```python
from build123d import *

# Parameters (mm, degrees)
F1_DEPTH = 7
F3_COUNT = 8
F3_ANGLE = 315


with BuildPart() as f1:
    # F0 (on Top) → F1 (new body)
    with BuildSketch(Plane.XY):
        with BuildLine():
            ThreePointArc((-1.4249641593, 5.3122007817), (-3.3475884696, -4.3639032343), (5.5, 0))
            ThreePointArc((5.5, 0), (4.3639032343, 3.3475884696), (1.4249641593, 5.3122007817))
            ThreePointArc((1.4249641593, 5.3122007817), (0, 5.5), (-1.4249641593, 5.3122007817))
        make_face()
        with BuildLine():
            ThreePointArc((-1.4249641593, 5.3122007817), (0, 5.5), (1.4249641593, 5.3122007817))
            ThreePointArc((1.4249641593, 5.3122007817), (1.5553934353, 6.597399257), (1.3891854213, 7.8784620241))
            ThreePointArc((1.3891854213, 7.8784620241), (0.9837129389, 8.990847184), (0.3543820184, 9.9937186965))
            ThreePointArc((0.3543820184, 9.9937186965), (0.1772188405, 9.9984295508), (0, 10))
            ThreePointArc((0, 10), (-0.1772188405, 9.9984295508), (-0.3543820184, 9.9937186965))
            ThreePointArc((-0.3543820184, 9.9937186965), (-0.3587995186, 9.9880877162), (-0.3632098505, 9.9824511198))
            ThreePointArc((-0.3632098505, 9.9824511198), (-0.9868539257, 8.9844162861), (-1.3891854213, 7.8784620241))
            ThreePointArc((-1.3891854213, 7.8784620241), (-1.5553934353, 6.597399257), (-1.4249641593, 5.3122007817))
        make_face()
    extrude(amount=F1_DEPTH)


with BuildPart() as f3_1:
    # F3: instance of F1
    add(f1.part.rotate(Axis((0, 0, 21.9664014876), (0, 0, -1)), 1 * F3_ANGLE / (F3_COUNT - 1)))


with BuildPart() as f3_2:
    # F3: instance of F1
    add(f1.part.rotate(Axis((0, 0, 21.9664014876), (0, 0, -1)), 2 * F3_ANGLE / (F3_COUNT - 1)))


with BuildPart() as f3_3:
    # F3: instance of F1
    add(f1.part.rotate(Axis((0, 0, 21.9664014876), (0, 0, -1)), 3 * F3_ANGLE / (F3_COUNT - 1)))


with BuildPart() as f3_4:
    # F3: instance of F1
    add(f1.part.rotate(Axis((0, 0, 21.9664014876), (0, 0, -1)), 4 * F3_ANGLE / (F3_COUNT - 1)))


with BuildPart() as f3_5:
    # F3: instance of F1
    add(f1.part.rotate(Axis((0, 0, 21.9664014876), (0, 0, -1)), 5 * F3_ANGLE / (F3_COUNT - 1)))


with BuildPart() as f3_6:
    # F3: instance of F1
    add(f1.part.rotate(Axis((0, 0, 21.9664014876), (0, 0, -1)), 6 * F3_ANGLE / (F3_COUNT - 1)))


with BuildPart() as f3_7:
    # F3: instance of F1
    add(f1.part.rotate(Axis((0, 0, 21.9664014876), (0, 0, -1)), 7 * F3_ANGLE / (F3_COUNT - 1)))


with BuildPart() as f3_6_1:
    add(f3_6.part)

    # F4: union F3_5, F3_4, F3_3, F3_2, F3_1, F1, F3_7
    add(f3_5.part)
    add(f3_4.part)
    add(f3_3.part)
    add(f3_2.part)
    add(f3_1.part)
    add(f1.part)
    add(f3_7.part)


solid = f3_6_1.part
```
Geometry check sheet. Reference: the model listing, model coordinates, mm. Round coordinates to 2 decimals unless told otherwise and drop trailing zeros. Order: outer loops, then holes, each group sorted by start corner. A loop starts at its lowest first (then second) coordinate and runs counter-clockwise, first axis right, second up. Notation, with made-up numbers: M 57.5,-26 L 61.5,-26 A36 cw 61.5,8 Z; hole C 60,4.25 d10. An arc over 180 degrees is marked long. Write item = value, one per line.
Q1. Scan lines: line 1 (Y direction, x = -6.25, z = 6.75); line 2 (Y direction, x = 5.5, z = 6.75). Record each from-to range of solid material in increasing order.
Answer block:
line_1 = -7.22 to -4.14, -1.55 to 1.55, 4.14 to 7.22
line_2 = -6.99 to -3.31, -1.46 to 1.46, 3.31 to 6.99
Q2. Depth check by flat-ended pin: pin 1 Ø4 at (x, z) = (-4.5, 5.5) entering from +Y; pin 2 Ø1.5 at (y, z) = (-1, 6) entering from -X; pin 3 Ø3 at (y, z) = (-4, 2) entering from +X. Enter the tip coordinate at first touch or a pass-through.
Answer block:
pin_1 = 7.27
pin_2 = -10
pin_3 = 6.99
Q3. Section check C-C (y = 2.5). Enter the section's corners in (x, z), plus the area to 3 significant figures.
Answer block:
outline = M -4.9,0 L 4.9,0 L 4.9,7 L -4.9,7 Z
area = 68.6 mm^2
Q4. Section check A-A (y = 5.75). Enter the section's corners in (x, z), plus the area to 3 significant figures.
Answer block:
outline = M -7.08,0 L -3.55,0 L -3.55,7 L -7.08,7 Z; M -1.5,0 L 1.5,0 L 1.5,7 L -1.5,7 Z; M 3.55,0 L 7.08,0 L 7.08,7 L 3.55,7 Z
area = 70.5 mm^2
Q5. Section check B-B (x = -5). Enter the section's corners in (y, z), plus the area to 4 significant figures.
Answer block:
outline = M -6.78,0 L -2.91,0 L -2.91,7 L -6.78,7 Z; M -2.29,0 L 2.29,0 L 2.29,7 L -2.29,7 Z; M 2.91,0 L 6.78,0 L 6.78,7 L 2.91,7 Z
area = 86.25 mm^2
Q6. Release check for a two-part mould opening along X. For faces 1 (the flat face through (0, 0, 0)), 2 (the cylindrical face through (-2.095, 5.085, 3.451)), 3 (the cylindrical face through (2.11, 5.08, 3.45)) record: released by +X, released by -X, zero draft, split by the parting line, or undercut.
Answer block:
face_1 = zero draft
face_2 = undercut
face_3 = undercut
Q7. Section check D-D (x = 2). Enter the section's corners in (y, z).
Answer block:
outline = M -5.12,0 L 5.12,0 L 5.12,7 L -5.12,7 Z
